from build123d import *

# Parameters (mm, degrees)
SKETCH_1_R          = 3
EXTRUDE_1_DEPTH     = 10
SKETCH_2_R          = 2.25
EXTRUDE_2_DEPTH     = 1.8
FILLET_2_R          = 2
CHAMFER_1_SIZE      = 0.5
CUT_EXTRUDE_1_DEPTH = 1.8


with BuildPart() as part:
    # 草图1 → 凸台-拉伸1 (new body)
    with BuildSketch(Plane(origin=(0, 0, 0), x_dir=(1, 0, 0), z_dir=(0, 1, 0))):
        with Locations(Location((0, 0, 0), (0, 0, 270))):
            Circle(SKETCH_1_R)
    extrude(amount=EXTRUDE_1_DEPTH)

    # 草图2 → 凸台-拉伸2 (add)
    with BuildSketch(Plane(origin=(0, 10, 0), x_dir=(1, 0, 0), z_dir=(0, 1, 0))):
        with Locations(Location((0, 0, 0), (0, 0, 270))):
            Circle(SKETCH_2_R)
    extrude(amount=EXTRUDE_2_DEPTH)

    # 圆角2
    # the kernel refuses this fillet: 2 mm, written as the material it takes off along each edge
    with BuildSketch(Plane(origin=(0, 11.8, 0), x_dir=(0, 0, 1), z_dir=(-1, 0, 0))) as fillet_2_piece_1:
        with BuildLine():
            CenterArc((0.260025126, -2), FILLET_2_R, 5.739170477, 84.260829523)
            Line((0.260025126, 0), (0.260025126, 0.04))
            Line((0.260025126, 0.04), (2.25, 0.04))
            Line((2.25, 0.04), (2.29, 0))
            ThreePointArc((2.29, 0), (2.29, -0.9), (2.289799497, -1.796))
            Line((2.289799497, -1.796), (2.25, -1.8))
        make_face()
    revolve(axis=Axis((0, 11.8, 0), (0, 1, 0)), mode=Mode.SUBTRACT)

    # 倒角1
    chamfer_1_edges = [part.edges().sort_by_distance(p)[0] for p in [
        (0, 0, -3),
    ]]
    chamfer(chamfer_1_edges, length=CHAMFER_1_SIZE)

    # 草图3 → 切除-拉伸1 (cut)
    with BuildSketch(Plane.XZ):
        Polygon((0, 1.808769012), (-1.566439914, 0.904384506), (-1.566439914, -0.904384506), (0, -1.808769012), (1.566439914, -0.904384506), (1.566439914, 0.904384506), align=None)
    extrude(amount=-CUT_EXTRUDE_1_DEPTH, mode=Mode.SUBTRACT)


solid = part.part
The listing builds one solid part. Answer for the finished solid, in the listing's coordinates (mm). Round coordinates to 2 decimals unless told otherwise and drop trailing zeros. Order: outer loops, then holes, each group sorted by start corner. A loop starts at its lowest first (then second) coordinate and runs counter-clockwise, first axis right, second up. Notation, with made-up numbers: (15.25, 77) -> (21.25, 77) arc R23 ccw to (21.25, 104) -> close; hole circle Ø11 at (2, 54). An arc over 180 degrees is marked (long way). Put each result on its own line as item: value.
Q1. Section A-A, the plane y = 1.25 is taken. Write down the section's boundary in (x, z).
Results list:
outline: circle Ø6 at (0, 0); hole (-1.57, -0.9) -> (0, -1.81) -> (1.57, -0.9) -> (1.57, 0.9) -> (0, 1.81) -> (-1.57, 0.9) -> close
Q2. Each of these flat-tipped pins is pushed along its axis until it touches: P1, Ø3, axis at x = 0.5, z = 2, coming from the +Y side; P2, Ø3, axis at x = -2.5, y = 9, coming from the -Z side. Where does it stop, or does it pass through?
Results list:
P1: y = 11.78
P2: z = -2.83
Q3. Determine the mould class of faces 1 (the cylindrical face through (0.9, 5.18, 2.86)), 2 (the flat face through (-2, 0, 0)), 3 (the flat face through (0.794, 0.887, 1.35)) for opening direction X: pulls with the +X half, pulls with the -X half, needs draft (parallel to the pull), parting line crosses it, or undercut.
Results list:
face 1: parting line crosses it
face 2: needs draft
face 3: undercut
Q4. Consider line 1 along Y through (x, z) = (2.4, 0.5); line 2 along X through (y, z) = (1, 1.15); line 3 along X through (y, z) = (1.25, -1.75). Determine where each line is inside the solid, lowest interval first.
Results list:
line 1: 0 to 10
line 2: -2.77 to -1.14, 1.14 to 2.77
line 3: -2.44 to -0.1, 0.1 to 2.44
